For this review, take the finished solid that the model builds, in its own axes (mm). Face numbers are marked on the shaded views. A direction names the side the tool comes from. Round coordinates to 2 decimals unless told otherwise and drop trailing zeros. Order: outer loops, then holes, each group sorted by start corner. A loop starts at its lowest first (then second) coordinate and runs counter-clockwise, first axis right, second up. Notation, with made-up numbers: (53, 78.5) -> (105, 78.5) arc R12 cw to (105, 87.5) -> close; hole circle Ø3 at (43.25, 42). An arc over 180 degrees is marked (long way). Answer in a Markdown table with one row per item.
```python
from build123d import *

# Parameters (mm, degrees)
SKETCH_1_W               = 20
SKETCH_1_H               = 20
SKETCH_1_W_2             = 16
SKETCH_1_H_2             = 16
EXTRUDE_1_DEPTH          = 83
SKETCH_2_R               = 2.2
CUT_EXTRUDE_1_DEPTH      = 83
SKETCH_3_R               = 6.5
CUT_EXTRUDE_2_DEPTH      = 3
SKETCH_4_R               = 2.2
CUT_EXTRUDE_3_DEPTH      = 1
CUT_EXTRUDE_3_DEPTH_BACK = 21
SKETCH_5_R               = 6.5
CUT_EXTRUDE_4_DEPTH      = 3


with BuildPart() as part:
    # ｽｹｯﾁ1 → ﾎﾞｽ - 押し出し1 (new body)
    with BuildSketch(Plane.XY):
        Rectangle(SKETCH_1_W, SKETCH_1_H)
        Rectangle(SKETCH_1_W_2, SKETCH_1_H_2, mode=Mode.SUBTRACT)
    extrude(amount=EXTRUDE_1_DEPTH)

    # ｽｹｯﾁ2 → ｶｯﾄ - 押し出し1 (cut)
    with BuildSketch(Plane(origin=(10, 0, 0), x_dir=(0, 0, -1), z_dir=(1, 0, 0))):
        with Locations((-66, 0)):
            Circle(SKETCH_2_R)
        with Locations((-17, 0)):
            Circle(SKETCH_2_R)
    extrude(amount=-CUT_EXTRUDE_1_DEPTH, mode=Mode.SUBTRACT)

    # ｽｹｯﾁ3 → ｶｯﾄ - 押し出し2 (cut)
    with BuildSketch(Plane(origin=(10, 0, 0), x_dir=(0, 0, -1), z_dir=(1, 0, 0))):
        with Locations((-66, 0)):
            Circle(SKETCH_3_R)
        with Locations((-17, 0)):
            Circle(SKETCH_3_R)
    extrude(amount=-CUT_EXTRUDE_2_DEPTH, mode=Mode.SUBTRACT)

    # ｽｹｯﾁ4 → ｶｯﾄ - 押し出し3 (cut, two sides)
    with BuildSketch(Plane.XZ.offset(10)) as cut_extrude_3_sk:
        with Locations((0, 56)):
            Circle(SKETCH_4_R)
        with Locations((0, 27)):
            Circle(SKETCH_4_R)
    extrude(amount=CUT_EXTRUDE_3_DEPTH, mode=Mode.SUBTRACT)
    extrude(cut_extrude_3_sk.sketch, amount=-CUT_EXTRUDE_3_DEPTH_BACK, mode=Mode.SUBTRACT)

    # ｽｹｯﾁ5 → ｶｯﾄ - 押し出し4 (cut)
    with BuildSketch(Plane(origin=(0, 10, 0), x_dir=(1, 0, 0), z_dir=(0, 1, 0))):
        with Locations((0, -56)):
            Circle(SKETCH_5_R)
        with Locations((0, -27)):
            Circle(SKETCH_5_R)
    extrude(amount=-CUT_EXTRUDE_4_DEPTH, mode=Mode.SUBTRACT)


solid = part.part
```
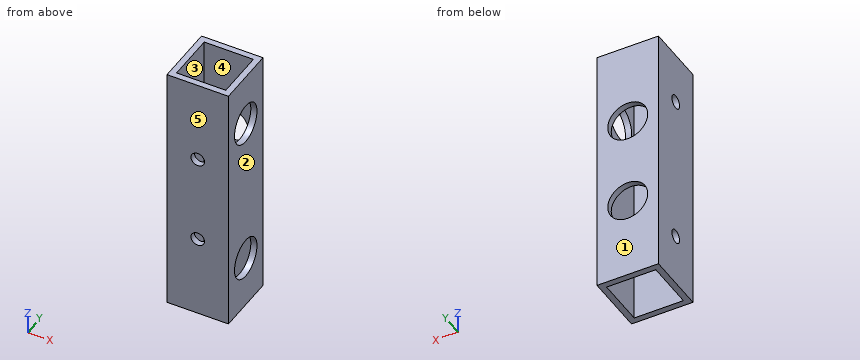
Q1. Take a section at A-A, the plane z = 74.5. Write out the cut boundary in (x, y), then the cut area to 3 significant figures.
Answer key:
| item | result |
|---|---|
| outline | (-10, -10) -> (10, -10) -> (10, 10) -> (-10, 10) -> close; hole (-8, -8) -> (8, -8) -> (8, 8) -> (-8, 8) -> close |
| area | 144 mm^2 |
Q2. To check wall thickness, follow probe 1 along Z at (x, y) = (0, 9.6); probe 2 along Y at (x, z) = (-9.2, 66); probe 3 along Y at (x, z) = (8.95, 17). State the ranges of each line that lie inside material, in increasing order.
Answer key:
| item | result |
|---|---|
| probe 1 | z = 0 to 20.5, 33.5 to 49.5, 62.5 to 83 |
| probe 2 | y = -10 to -2.2, 2.2 to 10 |
| probe 3 | y = -10 to -6.5, 6.5 to 10 |
Q3. Tool access review of the marked faces 4 and 5: name each direction out of +Z, -Z, +X, -X, +Y, -Y from which nothing blocks a thin tool from reaching the whole face with its end or side.
Answer key:
| item | result |
|---|---|
| face 4 | +Z, -Z |
| face 5 | +Z, -Z, +X, -X, -Y |
Q4. Take a section at D-D, the plane x = 0. Write out the cut boundary in (y, z), then the cut area to 3 significant figures.
Answer key:
| item | result |
|---|---|
| outline | (-10, 0) -> (-8, 0) -> (-8, 24.8) -> (-10, 24.8) -> close; (-10, 29.2) -> (-8, 29.2) -> (-8, 53.8) -> (-10, 53.8) -> close; (-10, 58.2) -> (-8, 58.2) -> (-8, 83) -> (-10, 83) -> close; (8, 0) -> (10, 0) -> (10, 20.5) -> (8, 20.5) -> close; (8, 33.5) -> (10, 33.5) -> (10, 49.5) -> (8, 49.5) -> close; (8, 62.5) -> (10, 62.5) -> (10, 83) -> (8, 83) -> close |
| area | 262 mm^2 |
Q5. Take a section at C-C, the plane z = 17. Write out the cut boundary in (x, y), then the cut area to 3 significant figures.
Answer key:
| item | result |
|---|---|
| outline | (-10, -10) -> (10, -10) -> (10, -6.5) -> (8, -6.5) -> (8, -8) -> (-8, -8) -> (-8, -2.2) -> (-10, -2.2) -> close; (-10, 2.2) -> (-8, 2.2) -> (-8, 8) -> (8, 8) -> (8, 6.5) -> (10, 6.5) -> (10, 10) -> (-10, 10) -> close |
| area | 109 mm^2 |
Q6. The part is to be moulded in two halves that separate along X. For the marked faces 1, 2 and 3, say which applies: +X half, -X half, draft (parallel to the pull), parting line (faces both ways), or undercut.
Answer key:
| item | result |
|---|---|
| face 1 | draft |
| face 2 | +X half |
| face 3 | undercut |
Q7. Clearance check with flat-ended pins moving along their axes: pin 1 Ø2 at (x, y) = (5.5, -6) entering from +Z; pin 2 Ø5 at (y, z) = (0, 66) entering from +X; pin 3 Ø5 at (x, z) = (0, 56) entering from +Y. State where each tip first meets the part, or that it passes through.
Answer key:
| item | result |
|---|---|
| pin 1 | passes through |
| pin 2 | stops at x = -8 |
| pin 3 | stops at y = -8 |
Q8. Take a section at B-B, the plane y = 0. Write out the cut boundary in (x, z).
Answer key:
| item | result |
|---|---|
| outline | (-10, 0) -> (-8, 0) -> (-8, 14.8) -> (-10, 14.8) -> close; (-10, 19.2) -> (-8, 19.2) -> (-8, 63.8) -> (-10, 63.8) -> close; (-10, 68.2) -> (-8, 68.2) -> (-8, 83) -> (-10, 83) -> close; (8, 0) -> (10, 0) -> (10, 10.5) -> (8, 10.5) -> close; (8, 23.5) -> (10, 23.5) -> (10, 59.5) -> (8, 59.5) -> close; (8, 72.5) -> (10, 72.5) -> (10, 83) -> (8, 83) -> close |
